```python
from build123d import *

# Parameters (mm, degrees)
BOSS_EXTRUDE1_DEPTH              = 3.175
F_11_64_0_17188_DIAMETER_HOLE1_D = 4.365752
FILLET1_R                        = 25.4


with BuildPart() as part:
    # Sketch1 → Boss-Extrude1 (new body)
    with BuildSketch(Plane(origin=(0, 0, 0), x_dir=(1, 0, 0), z_dir=(0, 1, 0))):
        with BuildLine():
            Line((-3.932886418, -2.685853807), (-25.4, -2.685853807))
            Line((-25.4, -2.685853807), (-28.085853807, -2.685853807))
            ThreePointArc((-28.085853807, -2.685853807), (-30.771707615, 0), (-28.085853807, 2.685853807))
            Line((-28.085853807, 2.685853807), (-25.4, 2.685853807))
            Line((-25.4, 2.685853807), (-3.932886418, 2.685853807))
            ThreePointArc((-3.932886418, 2.685853807), (4.7625, 0), (-3.932886418, -2.685853807))
        make_face()
    extrude(amount=BOSS_EXTRUDE1_DEPTH)

    # 11/64 (0.17188) Diameter Hole1 (through all)
    with Locations(Plane(origin=(0, 3.175, 0), x_dir=(1, 0, 0), z_dir=(0, 1, 0))):
        with Locations((0, 0)):
            Hole(F_11_64_0_17188_DIAMETER_HOLE1_D / 2)

    # Fillet1
    fillet1_edges = [part.edges().sort_by_distance(p)[0] for p in [
        (-3.932886418, 1.5875, -2.685853807),
        (-3.932886418, 1.5875, 2.685853807),
    ]]
    fillet(fillet1_edges, radius=FILLET1_R)


solid = part.part
```
Input: part model. Units: mm. Frame: model coordinates. A direction names the side the tool comes from. Round coordinates to 2 decimals unless told otherwise and drop trailing zeros. Loops run counter-clockwise (first coordinate to the right, second up) from the corner with the lowest first, then second, coordinate; pieces in that order, holes last.
1) Section query A-A on x = 0. Return the cut outline in (y, z) (1 decimal).
Ans:
outline: (0, -4.8) - (3.2, -4.8) - (3.2, -2.2) - (0, -2.2) - close; (0, 2.2) - (3.2, 2.2) - (3.2, 4.8) - (0, 4.8) - close
2) Section query C-C on y = 0.5. Return the cut outline in (x, z) (1 decimal), plus the area to 3 significant figures.
Ans:
outline: (-28.1, -2.7) - (-11, -2.7) arc R25.4 cw to (-1.7, -4.4) arc R4.8 ccw (long way) to (-1.7, 4.4) arc R25.4 cw to (-11, 2.7) - (-28.1, 2.7) arc R2.7 ccw to start; hole circle Ø4.4 at (0, 0)
area: 200 mm2
3) Pin query (flat end, axial travel): pin 1 (1.6 mm diameter, centred on x = -19, y = 1, fed in from +Z); pin 2 (1.5 mm diameter, centred on x = -21, y = 3, fed in from -Z). Return the tip coordinate at first contact, or that it passes through.
Ans:
pin 1: stops at z = 2.69
pin 2: stops at z = -2.69
4) Pull-direction query (Z, two-part tool) for faces 1 (the cylindrical face through (0.284, 1.565, -2.164)), 2 (the cylindrical face through (-30.77, 1.57, 0.06)), 3 (the flat face through (-13, 3.175, 0)), 4 (the flat face through (-20, 2, -2.686)); classes: released by +Z, released by -Z, zero draft, split by the parting line, or undercut.
Ans:
face 1: undercut
face 2: split by the parting line
face 3: zero draft
face 4: released by -Z
5) Section query D-D on x = -26. Return the cut outline in (y, z) (3 decimals).
Ans:
outline: (0, -2.686) - (3.175, -2.686) - (3.175, 2.686) - (0, 2.686) - close
6) Section query B-B on z = 0. Return the cut outline in (x, y) (1 decimal), plus the area to 3 significant figures.
Ans:
outline: (-30.8, 0) - (-2.2, 0) - (-2.2, 3.2) - (-30.8, 3.2) - close; (2.2, 0) - (4.8, 0) - (4.8, 3.2) - (2.2, 3.2) - close
area: 99.0 mm2
7) Material intervals for line 1 (Z direction, x = 0, y = 0.9); line 2 (Z direction, x = -0.5, y = 0.35); line 3 (X direction, y = 1.5, z = 0.75), sorted ascending.
Ans:
line 1: z = -4.76 to -2.18, 2.18 to 4.76
line 2: z = -4.74 to -2.12, 2.12 to 4.74
line 3: x = -30.66 to -2.05, 2.05 to 4.7
8) Set-up query: faces 5 (the flat face through (-19, 2, 2.686)), 6 (the cylindrical face through (-6.22, 1.61, -3.14)). Return all of +Z, -Z, +X, -X, +Y, -Y with unobstructed straight access to the full face (end or side cutting, diameter ignored); none if empty.
Ans:
face 5: +Z, -X, +Y, -Y
face 6: -Z, -X, +Y, -Y
